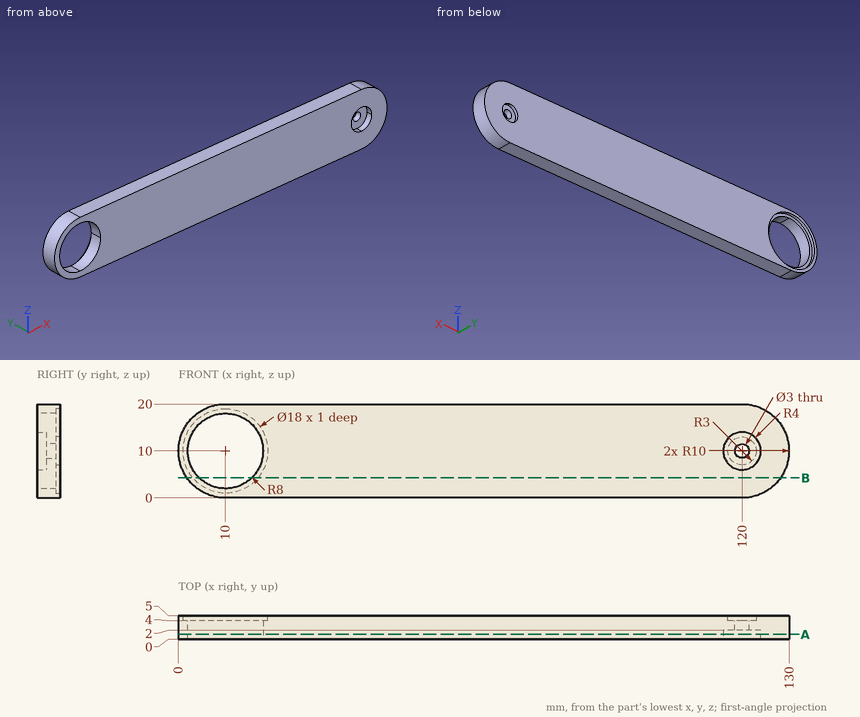
Geometry: see drawing. Coordinates: mm, zero at the bounding-box minimum. Give positions to 0.01 mm unless a question says otherwise; leave off trailing zeros. Loops run counter-clockwise (first coordinate to the right, second up) from the corner with the lowest first, then second, coordinate; pieces in that order, holes last. Notation, with made-up numbers: M 42.5,-4.75 L 93.5,-4.75 A15 ccw 93.5,1.25 Z; hole C 88.25,88.5 d3. An arc over 180 degrees is marked long. Answer as CSV lines item,"result". Start each with the question number.
1. Section A-A on y = 1.05. Return loops of the section in (x, z).
2. Line query: L1, parallel to X at y = 3.2, z = 10; L2, parallel to X at y = 4.8, z = 10; L3, parallel to Z at x = 120, y = 3.15. Output: solid intervals per line, ascending.
3. Pin query (flat end, axial travel): P1, Ø10, axis at x = 79, z = 9.5, coming from the -Y side; P2, Ø9, axis at x = 13.5, z = 9.5, coming from the +Y side; P3, Ø2.5, axis at x = 120, z = 10, coming from the -Y side; P4, Ø1.5, axis at y = 2.5, z = 8, coming from the -X side. Return the tip coordinate at first contact, or that it passes through.
4. Section B-B on z = 4.25. Return loops of the section in (x, y).
Computed values:
1,outline,"M 10,0 L 120,0 A10 ccw 120,20 L 10,20 A10 ccw Z; hole C 10,10 d16; hole C 120,10 d8"
2,L1,"x = 0 to 2, 18 to 118.5, 121.5 to 130"
2,L2,"x = 0 to 1, 19 to 117, 123 to 130"
2,L3,"z = 0 to 8.5, 11.5 to 20"
3,P1,"stops at y = 0"
3,P2,"stops at y = 4"
3,P3,"passes through"
3,P4,"stops at x = 0.08"
4,outline,"M 1.82,0 L 4.44,0 L 4.44,4 L 3.08,4 L 3.08,5 L 1.82,5 Z; M 15.56,0 L 128.18,0 L 128.18,5 L 16.92,5 L 16.92,4 L 15.56,4 Z"
